```python
from build123d import *

# Parameters (mm, degrees)
SKETCH1_W                = 28.575
SKETCH1_H                = 6.35
CUT_EXTRUDE1_DEPTH       = 7.35
CUT_EXTRUDE2_DEPTH       = 7.35
CUT_EXTRUDE3_DEPTH       = 7.35
CUT_EXTRUDE4_DEPTH       = 7.35
CUT_EXTRUDE5_DEPTH       = 7.35
CUT_EXTRUDE6_DEPTH       = 7.35
SKETCH8_R                = 15.24
BOSS_EXTRUDE1_DEPTH      = 41.275
M3_CLEARANCE_HOLE1_D     = 3.4544
M3_CLEARANCE_HOLE1_DEPTH = 47.625
CHAMFER1_SIZE            = 0.25
CHAMFER2_SIZE            = 1.5875
FILLET1_R                = 1


with BuildPart() as part:
    # Sketch1 → Revolve1 (revolve)
    with BuildSketch(Plane.XZ):
        with Locations((14.2875, 0)):
            Rectangle(SKETCH1_W, SKETCH1_H)
    revolve(axis=Axis((0, 0, 3.175), (0, 0, -1)))

    # Sketch2 → Cut-Extrude1 (cut, through all)
    with BuildSketch(Plane(origin=(0, 0, -3.175), x_dir=(-1, 0, 0), z_dir=(0, 0, -1))):
        with BuildLine():
            Line((13.824456468, 13.752614419), (18.067108165, 17.995266116))
            ThreePointArc((18.067108165, 17.995266116), (12.760996954, 22.077295051), (6.57534786, 24.637670355))
            Line((6.57534786, 24.637670355), (5.022432582, 18.842111637))
            ThreePointArc((5.022432582, 18.842111637), (9.760996476, 16.88114178), (13.824456468, 13.752614419))
        make_face()
    extrude(amount=-CUT_EXTRUDE1_DEPTH, mode=Mode.SUBTRACT)

    # Sketch3 → Cut-Extrude2 (cut, through all)
    with BuildSketch(Plane(origin=(0, 0, -3.175), x_dir=(-1, 0, 0), z_dir=(0, 0, -1))):
        with BuildLine():
            Line((-4.997885221, 18.848637704), (-6.550803522, 24.644207701))
            ThreePointArc((-6.550803522, 24.644207701), (-12.738999884, 22.089995065), (-18.049174487, 18.013253463))
            Line((-18.049174487, 18.013253463), (-13.806531048, 13.770610024))
            ThreePointArc((-13.806531048, 13.770610024), (-9.738999389, 16.893841804), (-4.997885221, 18.848637704))
        make_face()
    extrude(amount=-CUT_EXTRUDE2_DEPTH, mode=Mode.SUBTRACT)

    # Sketch4 → Cut-Extrude3 (cut, through all)
    with BuildSketch(Plane(origin=(0, 0, -3.175), x_dir=(-1, 0, 0), z_dir=(0, 0, -1))):
        with BuildLine():
            Line((-18.822341689, 5.096023285), (-24.617911686, 6.648941586))
            ThreePointArc((-24.617911686, 6.648941586), (-25.499996837, 0.012700014), (-24.624522347, -6.624416892))
            Line((-24.624522347, -6.624416892), (-18.82896363, -5.071501614))
            ThreePointArc((-18.82896363, -5.071501614), (-19.499995864, 0.012700024), (-18.822341689, 5.096023285))
        make_face()
    extrude(amount=-CUT_EXTRUDE3_DEPTH, mode=Mode.SUBTRACT)

    # Sketch5 → Cut-Extrude4 (cut, through all)
    with BuildSketch(Plane(origin=(0, 0, -3.175), x_dir=(-1, 0, 0), z_dir=(0, 0, -1))):
        with BuildLine():
            Line((-6.57534786, -24.637670355), (-5.022432582, -18.842111637))
            ThreePointArc((-5.022432582, -18.842111637), (-9.760996476, -16.88114178), (-13.824456468, -13.752614419))
            Line((-13.824456468, -13.752614419), (-18.067108165, -17.995266116))
            ThreePointArc((-18.067108165, -17.995266116), (-12.760996954, -22.077295051), (-6.57534786, -24.637670355))
        make_face()
    extrude(amount=-CUT_EXTRUDE4_DEPTH, mode=Mode.SUBTRACT)

    # Sketch6 → Cut-Extrude5 (cut, through all)
    with BuildSketch(Plane(origin=(0, 0, -3.175), x_dir=(-1, 0, 0), z_dir=(0, 0, -1))):
        with BuildLine():
            Line((18.049174487, -18.013253463), (13.806531048, -13.770610024))
            ThreePointArc((13.806531048, -13.770610024), (9.738999389, -16.893841804), (4.997885221, -18.848637704))
            Line((4.997885221, -18.848637704), (6.550803522, -24.644207701))
            ThreePointArc((6.550803522, -24.644207701), (12.738999884, -22.089995065), (18.049174487, -18.013253463))
        make_face()
    extrude(amount=-CUT_EXTRUDE5_DEPTH, mode=Mode.SUBTRACT)

    # Sketch7 → Cut-Extrude6 (cut, through all)
    with BuildSketch(Plane.XY.offset(3.175)):
        with BuildLine():
            Line((-18.82896363, 5.071501614), (-24.624522347, 6.624416892))
            ThreePointArc((-24.624522347, 6.624416892), (-25.499996837, -0.012700014), (-24.617911686, -6.648941586))
            Line((-24.617911686, -6.648941586), (-18.822341689, -5.096023285))
            ThreePointArc((-18.822341689, -5.096023285), (-19.499995864, -0.012700024), (-18.82896363, 5.071501614))
        make_face()
    extrude(amount=-CUT_EXTRUDE6_DEPTH, mode=Mode.SUBTRACT)

    # Sketch8 → Boss-Extrude1 (add)
    with BuildSketch(Plane.XY.offset(3.175)):
        Circle(SKETCH8_R)
    extrude(amount=BOSS_EXTRUDE1_DEPTH)

    # Sketch9 → Cut-Revolve1 (revolve, cut)
    with BuildSketch(Plane.XZ):
        Polygon((11.0998, 44.45), (0, 44.45), (0, -3.175), (11.0998, -3.175), (11.0998, 3.96875), (9.525, 3.96875), (9.525, 37.30625), (11.0998, 37.30625), align=None)
    revolve(axis=Axis((0, 0, 44.45), (0, 0, -1)), mode=Mode.SUBTRACT)

    # M3 Clearance Hole1
    with Locations(Plane(origin=(0, 0, -3.175), x_dir=(-1, 0, 0), z_dir=(0, 0, -1))):
        with Locations((-20.622229928, 11.90625), (-20.622229928, -11.90625), (0, -23.8125), (20.622229928, -11.90625), (20.622229928, 11.90625), (0, 23.8125)):
            Hole(M3_CLEARANCE_HOLE1_D / 2, depth=M3_CLEARANCE_HOLE1_DEPTH)

    # Chamfer1
    chamfer1_edges = [part.edges().sort_by_distance(p)[0] for p in [
        (-11.0998, 0, 44.45),
        (-11.0998, 0, -3.175),
        (-28.575, 0, -3.175),
        (-28.575, 0, 3.175),
    ]]
    chamfer(chamfer1_edges, length=CHAMFER1_SIZE)

    # Chamfer2
    chamfer2_edges = [part.edges().sort_by_distance(p)[0] for p in [
        (-15.24, 0, 44.45),
    ]]
    chamfer(chamfer2_edges, length=CHAMFER2_SIZE)

    # Fillet1
    fillet1_edges = [part.edges().sort_by_distance(p)[0] for p in [
        (-13.824456468, 13.752614419, 0),
        (-5.022432582, 18.842111637, 0),
        (-6.57534786, 24.637670355, 0),
        (-18.067108165, 17.995266116, 0),
        (4.997885221, 18.848637704, 0),
        (13.806531048, 13.770610024, 0),
        (18.049174487, 18.013253463, 0),
        (6.550803522, 24.644207701, 0),
        (18.822341689, 5.096023285, 0),
        (18.82896363, -5.071501614, 0),
        (24.624522347, -6.624416892, 0),
        (24.617911686, 6.648941586, 0),
        (6.57534786, -24.637670355, 0),
        (18.067108165, -17.995266116, 0),
        (13.824456468, -13.752614419, 0),
        (5.022432582, -18.842111637, 0),
        (-18.049174487, -18.013253463, 0),
        (-6.550803522, -24.644207701, 0),
        (-4.997885221, -18.848637704, 0),
        (-13.806531048, -13.770610024, 0),
        (-18.82896363, 5.071501614, 0),
        (-18.822341689, -5.096023285, 0),
        (-24.617911686, -6.648941586, 0),
        (-24.624522347, 6.624416892, 0),
    ]]
    fillet(fillet1_edges, radius=FILLET1_R)


solid = part.part
```
Geometry: final body of the model. Coordinates: model frame, mm. Round coordinates to 2 decimals unless told otherwise and drop trailing zeros. Order: outer loops, then holes, each group sorted by start corner. A loop starts at its lowest first (then second) coordinate and runs counter-clockwise, first axis right, second up. Notation, with made-up numbers: (26.25, 18) -> (65.25, 18) arc R30 cw to (65.25, 51) -> close; hole circle Ø7 at (16, -4). An arc over 180 degrees is marked (long way). Use one line per item in the form item = value. Start each with the question number.
1. Pin query (flat end, axial travel): pin 1 Ø4 at (x, y) = (-20.62, 11.91) entering from -Z (3 decimals); pin 2 Ø4 at (x, y) = (20.62, -11.91) entering from +Z (3 decimals); pin 3 Ø3 at (y, z) = (-3, 19) entering from +X; pin 4 Ø1.5 at (x, y) = (-4.5, 8) entering from +Z. Return the tip coordinate at first contact, or that it passes through.
2. Draft query along Y for faces 1 (the face through (-28.547, -1.256, 0.041)), 2 (the face through (17.62, 18.03, 0.04)), 3 (the face through (-5.76, -21.7, -0.04)), 4 (the face through (-12, 0, -3.175)). Return one class per face: pulls with the +Y half, pulls with the -Y half, needs draft (parallel to the pull), parting line crosses it, or undercut.
3. Cut plane A-A (x = 0). Count the separate pieces of the cut face and the enclosed holes in it, then the cut area to 3 significant figures.
4. Cut plane C-C (z = 7). Return the cut outline in (x, y) (3 decimals), then the cut area to 3 significant figures.
5. Line query: probe 1 along Y at (x, z) = (0, -0.25) (3 decimals); probe 2 along Z at (x, y) = (18, -2) (3 decimals); probe 3 along Y at (x, z) = (6.5, 26). Output: solid intervals per line, ascending.
Solution:
q1.pin_1 = -3.175
q1.pin_2 = 3.175
q1.pin_3 = 15.17
q1.pin_4 = 37.31
q2.face_1 = parting line crosses it
q2.face_2 = undercut
q2.face_3 = undercut
q2.face_4 = needs draft
q3.separate_pieces = 4
q3.enclosed_holes = 0
q3.area = 622 mm^2
q4.outline = circle Ø30.48 at (0, 0); hole circle Ø19.05 at (0, 0)
q4.area = 445 mm^2
q5.probe_1 = -28.575 to -25.54, -22.085 to -11.1, 11.1 to 22.085, 25.54 to 28.575
q5.probe_2 = -3.175 to 3.175
q5.probe_3 = -13.78 to -6.96, 6.96 to 13.78
